Source: CAD feature listing. Evaluate the final solid. Frame: model axes, mm. A direction names the side the tool comes from. Round coordinates to 2 decimals unless told otherwise and drop trailing zeros. Loops run counter-clockwise (first coordinate to the right, second up) from the corner with the lowest first, then second, coordinate; pieces in that order, holes last.
Item 1: Section query A-A on z = 0. Return loops of the section in (x, y) (3 decimals).
Item 2: Section query C-C on x = 1.5. Return loops of the section in (y, z) (3 decimals), then the cut area to 3 significant figures.
Item 3: First-contact query: P1, Ø2, axis at x = 3, z = 0, coming from the +Y side; P2, Ø2, axis at x = 11.5, z = 2, coming from the +Y side; P3, Ø1.2, axis at y = 0, z = 0, coming from the +X side; P4, Ø3, axis at x = 9, y = 2, coming from the -Z side. Flat tips, straight axial feed; report the tip coordinate or a pass-through.
Item 4: Section query B-B on x = 8.25. Return loops of the section in (y, z) (3 decimals), then the cut area to 3 significant figures.
Item 5: Access query for faces 1 (the flat face through (5.5, 1, -2)), 2 (the cylindrical face through (7.43, -0.54, 2.44)), 3 (the cylindrical face through (11, 0, 2)). Directions: +Z, -Z, +X, -X, +Y, -Y. A direction counts if a zero-diameter tool reaches every point of the face in a straight line with its end or side. Return the directions, or none.
Item 6: Ray query, L1, parallel to Y at x = 12, z = 0 (3 decimals); L2, parallel to Z at x = 8.75, y = 0 (3 decimals). Return the intervals inside material, ascending.
```python
from build123d import *

# Parameters (mm, degrees)
TROU_TARAUD_M2_52_D     = 2.05
TROU_TARAUD_M2_52_DEPTH = 7.35
TROU_TARAUD_M2_52_TIP   = 0.615882135
TROU_TARAUD_M2_51_D     = 2.05
CHANFREIN1_SIZE         = 0.3


with BuildPart() as part:
    # Esquisse1 → Révolution1 (revolve)
    with BuildSketch(Plane.XY):
        Polygon((0, 0), (0, 2), (5.5, 2), (5.5, 2.5), (9.3, 2.5), (9.3, 2), (13.8, 2), (13.8, 0), align=None)
    revolve(axis=Axis((13.8, 0, 0), (-1, 0, 0)))

    # Trou taraudé M2.52
    with Locations(Plane.ZY):
        with Locations((0, 0)):
            Hole(TROU_TARAUD_M2_52_D / 2, depth=TROU_TARAUD_M2_52_DEPTH)
            with Locations((0, 0, -(TROU_TARAUD_M2_52_DEPTH + TROU_TARAUD_M2_52_TIP / 2))):  # 118° drill point
                Cone(0, TROU_TARAUD_M2_52_D / 2, TROU_TARAUD_M2_52_TIP, mode=Mode.SUBTRACT)

    # Trou taraudé M2.51 (through all)
    with Locations(Plane(origin=(13.8, 0, 0), x_dir=(0, 0, -1), z_dir=(1, 0, 0))):
        with Locations((0, 0)):
            Hole(TROU_TARAUD_M2_51_D / 2)

    # Chanfrein1
    chanfrein1_edges = [part.edges().sort_by_distance(p)[0] for p in [
        (0, -2, 0),
        (13.8, -2, 0),
    ]]
    chamfer(chanfrein1_edges, length=CHANFREIN1_SIZE)


solid = part.part
```
Data:
1. outline: (0, -1.7) - (0.3, -2) - (5.5, -2) - (5.5, -2.5) - (9.3, -2.5) - (9.3, -2) - (13.5, -2) - (13.8, -1.7) - (13.8, -1.025) - (0, -1.025) - close; (0, 1.025) - (13.8, 1.025) - (13.8, 1.7) - (13.5, 2) - (9.3, 2) - (9.3, 2.5) - (5.5, 2.5) - (5.5, 2) - (0.3, 2) - (0, 1.7) - close
2. outline: circle Ø4 at (0, 0); hole circle Ø2.05 at (0, 0)
2. area: 9.27 mm2
3. P1: stops at y = 2
3. P2: stops at y = 1.73
3. P3: passes through
3. P4: stops at z = -2.45
4. outline: circle Ø5 at (0, 0); hole circle Ø2.05 at (0, 0)
4. area: 16.3 mm2
5. face 1: -X
5. face 2: +X, -X
5. face 3: +X
6. L1: y = -2 to -1.025, 1.025 to 2
6. L2: z = -2.5 to -1.025, 1.025 to 2.5
